Geometry check sheet. Reference: the model listing, model coordinates, mm. Face numbers are marked on the shaded views. A direction names the side the tool comes from. Coordinates: 2 decimals unless noted, no trailing zeros. Write each loop counter-clockwise with the first axis right and the second up, starting at its lowest first coordinate (ties: lowest second). Pieces come first, ordered by that corner, then holes. Notation, with made-up numbers: (-19, 86.5) -> (-15, 86.5) arc R8 ccw to (-15, 94.5) -> close; hole circle Ø4 at (-26, 74). An arc over 180 degrees is marked (long way). One line per question, with ' | ' between items.
```python
from build123d import *

# Parameters (mm, degrees)
SKETCH1_W            = 12.0015
SKETCH1_H            = 9.9822
BOSS_EXTRUDE4_DEPTH  = 9.0678
BOSS_EXTRUDE5_DEPTH  = 15.1003
SKETCH4_R            = 2.00025
BOSS_EXTRUDE9_DEPTH  = 1.016
BOSS_EXTRUDE10_DEPTH = 9.0678
SKETCH6_R            = 2.5146
BOSS_EXTRUDE11_DEPTH = 0.889
SKETCH7_R            = 0.508
BOSS_EXTRUDE12_DEPTH = 4.3053


with BuildPart() as part:
    # Sketch1 → Boss-Extrude4 (new body)
    with BuildSketch(Plane.XY):
        with Locations((11.58762082, -8.953965436)):
            Rectangle(SKETCH1_W, SKETCH1_H)
    extrude(amount=BOSS_EXTRUDE4_DEPTH)

    # Sketch3 → Boss-Extrude5 (add)
    with BuildSketch(Plane(origin=(0, 0, 0), x_dir=(-1, 0, 0), z_dir=(0, 0, -1))):
        with BuildLine():
            Line((-14.919017466, -3.924765436), (-8.256224175, -3.924765436))
            ThreePointArc((-8.256224175, -3.924765436), (-5.55512082, -8.953965436), (-8.256224175, -13.983165436))
            Line((-8.256224175, -13.983165436), (-14.919017466, -13.983165436))
            ThreePointArc((-14.919017466, -13.983165436), (-17.62012082, -8.953965436), (-14.919017466, -3.924765436))
        make_face()
    extrude(amount=BOSS_EXTRUDE5_DEPTH)

    # Sketch4 → Boss-Extrude9 (add)
    with BuildSketch(Plane.XY.offset(9.0678)):
        with Locations((11.58762082, -8.953965436)):
            Circle(SKETCH4_R)
    extrude(amount=BOSS_EXTRUDE9_DEPTH)

    # Sketch5 → Boss-Extrude10 (add)
    with BuildSketch(Plane.XY.offset(10.0838)):
        with BuildLine():
            Line((10.494618208, -7.926665436), (12.680623432, -7.926665436))
            ThreePointArc((12.680623432, -7.926665436), (11.58762082, -10.453965436), (10.494618208, -7.926665436))
        make_face()
    extrude(amount=BOSS_EXTRUDE10_DEPTH)

    # Sketch6 → Boss-Extrude11 (add)
    with BuildSketch(Plane(origin=(0, 0, -15.1003), x_dir=(-1, 0, 0), z_dir=(0, 0, -1))):
        with Locations((-11.58762082, -8.953965436)):
            Circle(SKETCH6_R)
    extrude(amount=BOSS_EXTRUDE11_DEPTH)

    # Sketch7 → Boss-Extrude12 (add)
    with BuildSketch(Plane(origin=(0, 0, -15.9893), x_dir=(-1, 0, 0), z_dir=(0, 0, -1))):
        with Locations((-11.58762082, -8.953965436)):
            Circle(SKETCH7_R)
    extrude(amount=BOSS_EXTRUDE12_DEPTH)


solid = part.part
```
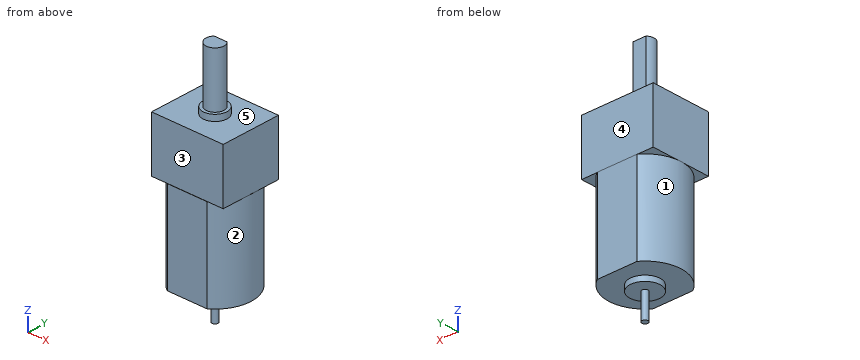
(1) Depth check by flat-ended pin: P1, Ø3, axis at x = 17, y = -5.5, coming from the -Z side; P2, Ø4.5, axis at x = 14, z = 3, coming from the -Y side; P3, Ø2.5, axis at x = 12.5, z = 5, coming from the +Y side. Enter the tip coordinate at first touch or a pass-through.
Answers below:
P1: stops at z = -15.1 | P2: stops at y = -13.95 | P3: stops at y = -3.96
(2) Material ranges on line 1 (Z direction, x = 13.5, y = -6); line 2 (Y direction, x = 7.75, z = 2); line 3 (X direction, y = -7, z = 2.5), recorded low to high.
Answers below:
line 1: z = -15.1 to 9.07 | line 2: y = -13.95 to -3.96 | line 3: x = 5.59 to 17.59
(3) Cross-section at D-D (y = -7.5). Record the cut outline in (x, z).
Answers below:
outline: (5.59, 0) -> (5.73, 0) -> (5.73, -15.1) -> (9.54, -15.1) -> (9.54, -15.99) -> (13.64, -15.99) -> (13.64, -15.1) -> (17.44, -15.1) -> (17.44, 0) -> (17.59, 0) -> (17.59, 9.07) -> (12.96, 9.07) -> (12.96, 10.08) -> (10.21, 10.08) -> (10.21, 9.07) -> (5.59, 9.07) -> close
(4) Cross-section at C-C (z = -2.5). Record the cut outline in (x, y) (1 decimal), plus the area to 3 significant figures.
Answers below:
outline: (8.3, -14) -> (14.9, -14) arc R6 ccw to (14.9, -3.9) -> (8.3, -3.9) arc R6 ccw to start | area: 105 mm²
(5) Cross-section at A-A (x = 7). Record the cut outline in (y, z), plus the area to 3 significant figures.
Answers below:
outline: (-13.95, 0) -> (-12.87, 0) -> (-12.87, -15.1) -> (-5.04, -15.1) -> (-5.04, 0) -> (-3.96, 0) -> (-3.96, 9.07) -> (-13.95, 9.07) -> close | area: 209 mm²
(6) Tool access check on the marked faces 1, 2, 3, 4 and 5. Record the directions out of +Z, -Z, +X, -X, +Y, -Y that give a thin tool (end or side, any length) a straight path to the whole face; none if there is none.
Answers below:
face 1: -Z, -X | face 2: -Z, +X | face 3: +Z, +X, -X, -Y | face 4: +Z, +X, -X, +Y | face 5: +Z
(7) Cross-section at B-B (y = -13). Record the cut outline in (x, z).
Answers below:
outline: (5.59, 0) -> (7.11, 0) -> (7.11, -15.1) -> (16.06, -15.1) -> (16.06, 0) -> (17.59, 0) -> (17.59, 9.07) -> (5.59, 9.07) -> close
